```python
from build123d import *

# Parameters (mm, degrees)
F1_DEPTH = 8
F2_R     = 1.5
F3_W     = 3
F3_H     = 3
F4_DEPTH = 9
F5_R     = 0.75


with BuildPart() as f1:
    # F0 (on Top) → F1 (new body)
    with BuildSketch(Plane.XY):
        Polygon((0, 6), (0, 0), (30, 0), (30, 10), align=None)
    extrude(amount=F1_DEPTH)

    # F2
    f2_edges = [f1.edges().sort_by_distance(p)[0] for p in [
        (30, 0, 4),
        (0, 0, 4),
        (30, 10, 4),
        (0, 6, 4),
    ]]
    fillet(f2_edges, radius=F2_R)


with BuildPart() as f4:
    # F3 (on Top) → F4 (new body)
    with BuildSketch(Plane.XY):
        Rectangle(F3_W, F3_H)
    extrude(amount=F4_DEPTH)

    # F5
    f5_edges = [f4.edges().sort_by_distance(p)[0] for p in [
        (1.5, -1.5, 4.5),
        (-1.5, -1.5, 4.5),
        (1.5, 1.5, 4.5),
        (-1.5, 1.5, 4.5),
    ]]
    fillet(f5_edges, radius=F5_R)


with BuildPart() as f4_1:
    # F6: moved
    add(f4.part.moved(Location((25, 4, 0))))


with BuildPart() as f7_1:
    # F7: copy of F4
    add(f4_1.part)


with BuildPart() as f7_1_1:
    # F8: moved
    add(f7_1.part.moved(Location((-10, 0, 0))))


with BuildPart() as f9_1:
    # F9: copy of F7_1
    add(f7_1_1.part)


with BuildPart() as f9_1_1:
    # F10: moved
    add(f9_1.part.moved(Location((-10, 0, 0))))


with BuildPart() as f4_2:
    # F11: moved
    add(f4_1.part.moved(Location((0, -1, 0))))


with BuildPart() as f7_1_2:
    # F11: moved
    add(f7_1_1.part.moved(Location((0, -1, 0))))


with BuildPart() as f9_1_2:
    # F11: moved
    add(f9_1_1.part.moved(Location((0, -1, 0))))


with BuildPart() as f1_1:
    add(f1.part)

    # F12: cut F7_1, F4, F9_1
    add(f7_1_2.part, mode=Mode.SUBTRACT)
    add(f4_2.part, mode=Mode.SUBTRACT)
    add(f9_1_2.part, mode=Mode.SUBTRACT)


solid = f1_1.part
```
Here's how the part is built. I have some questions about the finished solid (model axes, mm). A direction names the side the tool comes from. Coordinates: 2 decimals unless noted, no trailing zeros. Loops run counter-clockwise (first coordinate to the right, second up) from the corner with the lowest first, then second, coordinate; pieces in that order, holes last. Notation, with made-up numbers: M -0.5,-21.75 L 30.5,-21.75 A34 cw 30.5,11.25 Z; hole C 61.5,-31 d11. An arc over 180 degrees is marked long. One line per item, written item: value.
1. On a 3-axis mill with a long thin cutter (end or side, diameter ignored), from which of +Z, -Z, +X, -X, +Y, -Y can I reach the whole of each face in a straight line? I mean faces 1 (the flat face through (15, 5, 8)), 2 (the flat face through (23.5, 3, 4)). Say none if no direction works.
Geometry says:
face 1: +Z, +X, -X, +Y, -Y
face 2: +Z, -Z
2. Please list where these lines run through material, in increasing order: probe 1 along X at (y, z) = (3.75, 1); probe 2 along Y at (x, z) = (13.75, 3.75); probe 3 along Y at (x, z) = (24.75, 7.25).
Geometry says:
probe 1: x = 0 to 3.5, 6.5 to 13.5, 16.5 to 23.5, 26.5 to 30
probe 2: y = 0 to 1.69, 4.31 to 7.83
probe 3: y = 0 to 1.5, 4.5 to 9.3
3. Will these pins go through, and if not, where does the flat tip stop? pin 1 Ø1.6 at (x, z) = (25, 5.5) entering from +Y; pin 2 Ø1 at (x, y) = (16, 4) entering from -Z; pin 3 Ø2 at (x, z) = (4.5, 1.5) entering from +Y; pin 4 Ø0.8 at (x, z) = (15, 6) entering from +Y.
Geometry says:
pin 1: stops at y = 9.44
pin 2: stops at z = 0
pin 3: stops at y = 6.73
pin 4: stops at y = 8.05
4. Imagine slicing it at C-C (x = 11.25). List the corners of the cut face in (y, z) for me, and give its area (3 significant figures).
Geometry says:
outline: M 0,0 L 7.5,0 L 7.5,8 L 0,8 Z
area: 60.0 mm2
5. Imagine slicing it at A-A (y = 2.75). List the corners of the cut face in (x, z) for me.
Geometry says:
outline: M 0,0 L 3.5,0 L 3.5,8 L 0,8 Z; M 6.5,0 L 13.5,0 L 13.5,8 L 6.5,8 Z; M 16.5,0 L 23.5,0 L 23.5,8 L 16.5,8 Z; M 26.5,0 L 30,0 L 30,8 L 26.5,8 Z
6. Imagine slicing it at B-B (z = 3). State how many separate pieces and enclosed holes the cut face has, and give its area (3 significant figures).
Geometry says:
separate pieces: 1
enclosed holes: 3
area: 212 mm2
7. Thinking about a two-plate mould opening in Y: for faces 3 (the flat face through (26.5, 3, 4)), 4 (the cylindrical face through (0.43, 0.45, 4.06)), 5 (the cylindrical face through (0.36, 5.66, 4.06)), which applies, +Y half, -Y half, draft (parallel to the pull), parting line (faces both ways), or undercut?
Geometry says:
face 3: undercut
face 4: -Y half
face 5: +Y half
